```python
from build123d import *

# Parameters (mm, degrees)
SKETCH1_W                    = 1420
SKETCH1_H                    = 125
BASE_FLANGE1_DEPTH           = 4
EDGE_FLANGE1_STRIP_W         = 28
EDGE_FLANGE1_STRIP_H         = 4
EDGE_FLANGE1_STRIP_CUT_DEPTH = 1420
EDGE_FLANGE1_DEPTH           = 1420
EDGE_FLANGE2_STRIP_W         = 28
EDGE_FLANGE2_STRIP_H         = 4
EDGE_FLANGE2_STRIP_CUT_DEPTH = 1420
EDGE_FLANGE2_DEPTH           = 1420


# Sheet-metal steps are written as plain solids
with BuildPart() as part:
    # Sketch1 → Base-Flange1 (new body)
    with BuildSketch(Plane.XY):
        with Locations((-226.8723099, 44.386657102)):
            Rectangle(SKETCH1_W, SKETCH1_H)
    extrude(amount=-BASE_FLANGE1_DEPTH)

    # Edge-Flange1 strip (across the edge) → Edge-Flange1 strip cut (cut)
    with BuildSketch(Plane(origin=(483.1276901, 106.886657102, 0), x_dir=(0, -1, 0), z_dir=(-1, 0, 0))):
        with Locations((-4, -2)):
            Rectangle(EDGE_FLANGE1_STRIP_W, EDGE_FLANGE1_STRIP_H)
    extrude(amount=EDGE_FLANGE1_STRIP_CUT_DEPTH, mode=Mode.SUBTRACT)

    # Edge-Flange1 section (across the edge) → Edge-Flange1 (add)
    with BuildSketch(Plane(origin=(483.1276901, 106.886657102, 0), x_dir=(0, -1, 0), z_dir=(-1, 0, 0))):
        with BuildLine():
            Line((0, 6), (0, 58))
            Line((0, 58), (4, 58))
            Line((4, 58), (4, 6))
            ThreePointArc((4, 6), (5.757359313, 1.757359313), (10, 0))
            Line((10, 0), (10, -4))
            ThreePointArc((10, -4), (2.928932188, -1.071067812), (0, 6))
        make_face()
    extrude(amount=EDGE_FLANGE1_DEPTH)

    # Edge-Flange2 strip (across the edge) → Edge-Flange2 strip cut (cut)
    with BuildSketch(Plane(origin=(-936.8723099, -18.113342898, 0), x_dir=(0, 1, 0), z_dir=(1, 0, 0))):
        with Locations((-4, -2)):
            Rectangle(EDGE_FLANGE2_STRIP_W, EDGE_FLANGE2_STRIP_H)
    extrude(amount=EDGE_FLANGE2_STRIP_CUT_DEPTH, mode=Mode.SUBTRACT)

    # Edge-Flange2 section (across the edge) → Edge-Flange2 (add)
    with BuildSketch(Plane(origin=(-936.8723099, -18.113342898, 0), x_dir=(0, 1, 0), z_dir=(1, 0, 0))):
        with BuildLine():
            Line((0, 6), (0, 58))
            Line((0, 58), (4, 58))
            Line((4, 58), (4, 6))
            ThreePointArc((4, 6), (5.757359313, 1.757359313), (10, 0))
            Line((10, 0), (10, -4))
            ThreePointArc((10, -4), (2.928932188, -1.071067812), (0, 6))
        make_face()
    extrude(amount=EDGE_FLANGE2_DEPTH)


solid = part.part
```
Can you work these out from the model? Positions are in its coordinate system, mm. A direction names the side the tool comes from. Round coordinates to 2 decimals unless told otherwise and drop trailing zeros. Loops run counter-clockwise (first coordinate to the right, second up) from the corner with the lowest first, then second, coordinate; pieces in that order, holes last. Notation, with made-up numbers: M -0.5,-39.5 L 57.5,-39.5 A27 ccw 57.5,-3.5 Z; hole C 54,43.5 d10. An arc over 180 degrees is marked long. Answer as a JSON object with one key per item and string values. Group by question number.
Q1. Imagine slicing it at A-A, the plane z = 27.5. Please give me the cut outline in (x, y), then the cut area to 3 significant figures.
Q2. Imagine slicing it at C-C, the plane y = 8. Please give me the cut outline in (x, z), then the cut area to 3 significant figures.
Q3. On a 3-axis mill with a long thin cutter (end or side, diameter ignored), from which of +Z, -Z, +X, -X, +Y, -Y can I reach the whole of each face in a straight line? I mean faces 4 (the flat face through (-936.872, 44.7, -0.4)), 5 (the flat face through (-237, 45, 0)). Say none if no direction works.
Q4. We'd pull the mould along Y, two halves only. Please class faces 1 (the flat face through (-237, -18.113, 32)), 2 (the flat face through (483.128, 44.7, -0.4)), 3 (the flat face through (-217, 102.887, 32)): +Y half, -Y half, draft (parallel to the pull), parting line (faces both ways), or undercut.
Q5. Please list where these lines run through material, in increasing order: L1, parallel to Y at x = 105, z = 52; L2, parallel to Z at x = -469, y = 41.5; L3, parallel to Z at x = -843, y = -10.
Q6. Will this pin go through, and if not, where does the flat tip stop? pin 1 (10 mm diameter, centred on x = 42.5, y = 3, fed in from +Z).
Q7. Imagine slicing it at B-B, the plane x = 132. Please give me the cut outline in (y, z), then the cut area to 3 significant figures.
Findings:
{
 "1": {"outline": "M -936.87,-18.11 L 483.13,-18.11 L 483.13,-14.11 L -936.87,-14.11 Z; M -936.87,102.89 L 483.13,102.89 L 483.13,106.89 L -936.87,106.89 Z", "area": "11,400 mm2"},
 "2": {"outline": "M -936.87,-4 L 483.13,-4 L 483.13,0 L -936.87,0 Z", "area": "5,680 mm2"},
 "3": {"face 4": "+Z, -Z, -X, +Y, -Y", "face 5": "+Z, +X, -X"},
 "4": {"face 1": "-Y half", "face 2": "draft", "face 3": "undercut"},
 "5": {"L1": "y = -18.11 to -14.11, 102.89 to 106.89", "L2": "z = -4 to 0", "L3": "z = -3.82 to 0.3"},
 "6": {"pin 1": "stops at z = 0"},
 "7": {"outline": "M -18.11,6 A10 ccw -8.11,-4 L 96.89,-4 A10 ccw 106.89,6 L 106.89,58 L 102.89,58 L 102.89,6 A6 cw 96.89,0 L -8.11,0 A6 cw -14.11,6 L -14.11,58 L -18.11,58 Z", "area": "937 mm2"}
}
